Input: part model. Units: mm. Frame: model coordinates. A direction names the side the tool comes from. Coordinates: 2 decimals unless noted, no trailing zeros. Order: outer loops, then holes, each group sorted by start corner. A loop starts at its lowest first (then second) coordinate and runs counter-clockwise, first axis right, second up.
Autodesk Inventor part; units mm, degrees
ref_plane "YZ Plane" through (0, 0, 0) normal (1, 0, 0) x (0, 1, 0)
ref_plane "XZ Plane" through (0, 0, 0) normal (0, 1, 0) x (-1, 0, 0)
ref_plane "XY Plane" through (0, 0, 0) normal (0, 0, 1) x (1, 0, 0)
sketch "Sketch1" plane through (0, 0, 0) normal (0, 1, 0) x (-1, 0, 0)
  circle A0 centre (0, 0) radius 1.5
  dimension "d0" = 3
extrude "Extrusion1" add sketch "Sketch1" along normal blind 5
sketch "Sketch2" plane through (0, 5, 0) normal (0, 1, 0) x (1, 0, 0)
  circle A0 centre (0, 0) radius 1.5
  circle A1 centre (0, 0) radius 3.25
  dimension "d3" = 6.5
extrude "Extrusion2" add sketch "Sketch2" along normal blind 15 contours A0 | A1
sketch "Sketch3" plane through (0, 20, 0) normal (0, 1, 0) x (1, 0, 0)
  circle A0 centre (0, 0) radius 1.5
  circle A1 centre (0, 0) radius 1.6
  dimension "d6" = 3.2
extrude "Extrusion3" cut sketch "Sketch3" against normal blind 2.5 contours A0 | A1
properties part number "ControlPanel_shortStands"
Item 1: Cut plane D-D on y = 15.25. Return loops of the section in (x, z), then the cut area to 3 significant figures.
Response values:
outline: circle Ø6.5 at (0, 0)
area: 33.2 mm2
Item 2: Cut plane A-A on z = 0. Return loops of the section in (x, y).
Response values:
outline: (-3.25, 5) - (-1.5, 5) - (-1.5, 0) - (1.5, 0) - (1.5, 5) - (3.25, 5) - (3.25, 20) - (1.6, 20) - (1.6, 17.5) - (-1.6, 17.5) - (-1.6, 20) - (-3.25, 20) - close
Item 3: Pin query (flat end, axial travel): pin 1 Ø1.6 at (x, z) = (-0.5, 0) entering from +Y; pin 2 Ø1 at (x, z) = (-2.5, -1.5) entering from -Y. Return the tip coordinate at first contact, or that it passes through.
Response values:
pin 1: stops at y = 17.5
pin 2: stops at y = 5
Item 4: Ray query, probe 1 along X at (y, z) = (18.1, 0); probe 2 along Y at (x, z) = (0.5, -2.75). Return the intervals inside material, ascending.
Response values:
probe 1: x = -3.25 to -1.6, 1.6 to 3.25
probe 2: y = 5 to 20
Item 5: Access query for faces 1 (the face through (-2.579, 12.395, -1.978)), 2 (the face through (0, 17.5, 0)), 3 (the face through (0.7, 5, -1.5)). Directions: +Z, -Z, +X, -X, +Y, -Y. A direction counts if a zero-diameter tool reaches every point of the face in a straight line with its end or side. Return the directions, or none.
Response values:
face 1: +Y, -Y
face 2: +Y
face 3: -Y
Item 6: Cut plane C-C on y = 3.25. Return loops of the section in (x, z), then the cut area to 3 significant figures.
Response values:
outline: circle Ø3 at (0, 0)
area: 7.07 mm2
Item 7: Cut plane B-B on x = 0. Return loops of the section in (y, z).
Response values:
outline: (0, -1.5) - (5, -1.5) - (5, -3.25) - (20, -3.25) - (20, -1.6) - (17.5, -1.6) - (17.5, 1.6) - (20, 1.6) - (20, 3.25) - (5, 3.25) - (5, 1.5) - (0, 1.5) - close
Item 8: Draft query along X for faces 4 (the face through (-1.27, 18.77, 0.97)), 5 (the face through (0, 0, 0)), 6 (the face through (1.5, 2.46, -0.07)). Return one class per face: pulls with the +X half, pulls with the -X half, needs draft (parallel to the pull), parting line crosses it, or undercut.
Response values:
face 4: undercut
face 5: needs draft
face 6: parting line crosses it
